```python
from build123d import *

# Parameters (mm, degrees)
F0_W     = 20.769432
F0_H     = 34.9758
F1_DEPTH = 2.54


with BuildPart() as f1:
    # F0 (on Front) → F1 (new body)
    with BuildSketch(Plane.XZ):
        Polygon((-12.7, 0), (0, 0), (12.7, 0), (12.7, 9.4996), (-12.7, 9.4996), align=None)
        Polygon((-12.7, 18.4404), (-12.7, 9.4996), (12.7, 9.4996), (12.7, 18.4404), (11.725585, 18.4404), (-11.725585, 18.4404), align=None)
        Polygon((-11.725585, 28.448), (-11.725585, 18.4404), (11.725585, 18.4404), (11.725585, 28.448), (10.384716, 28.448), (-10.384716, 28.448), align=None)
        with Locations((0, 45.9359)):
            Rectangle(F0_W, F0_H)
    extrude(amount=-F1_DEPTH)


solid = f1.part
```
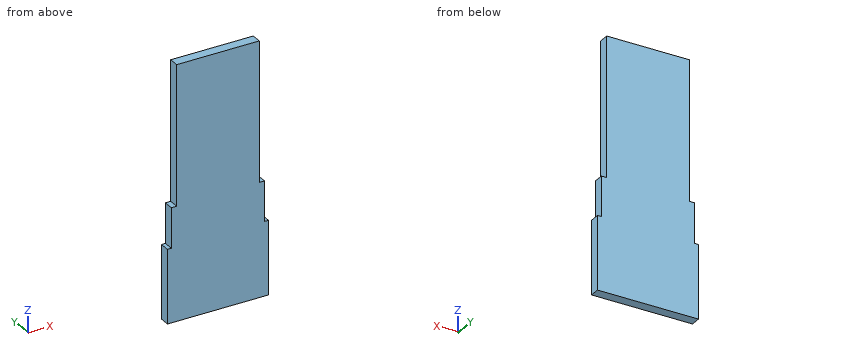
Verification items for the finished model (mm, model axes). Give positions to 0.01 mm unless a question says otherwise; leave off trailing zeros. Loops run counter-clockwise (first coordinate to the right, second up) from the corner with the lowest first, then second, coordinate; pieces in that order, holes last.
1. Section check A-A, the plane y = 1.1. Enter the section's corners in (x, z).
2. Thickness scan on line 1 (Z direction, x = 11.25, y = 0.2); line 2 (X direction, y = 1.25, z = 58.5); line 3 (X direction, y = 1.6, z = 22). Record the ranges inside material, lowest first.
3. Section check B-B, the plane z = 30.5. Enter the section's corners in (x, y), then the cut area to 3 significant figures.
4. Go/stop test with flat-tipped pins: pin 1 Ø1.1 at (x, y) = (-11, 2) entering from +Z; pin 2 Ø1.5 at (x, y) = (11, 1.5) entering from +Z; pin 3 Ø1.3 at (y, z) = (1, 25) entering from -X; pin 4 Ø1.3 at (y, z) = (1, 42) entering from -X. Record where each tip stops, or that it passes through.
Geometry says:
1. outline: (-12.7, 0) - (12.7, 0) - (12.7, 18.44) - (11.73, 18.44) - (11.73, 28.45) - (10.38, 28.45) - (10.38, 63.42) - (-10.38, 63.42) - (-10.38, 28.45) - (-11.73, 28.45) - (-11.73, 18.44) - (-12.7, 18.44) - close
2. line 1: z = 0 to 28.45
2. line 2: x = -10.38 to 10.38
2. line 3: x = -11.73 to 11.73
3. outline: (-10.38, 0) - (10.38, 0) - (10.38, 2.54) - (-10.38, 2.54) - close
3. area: 52.8 mm2
4. pin 1: stops at z = 28.45
4. pin 2: stops at z = 63.42
4. pin 3: stops at x = -11.73
4. pin 4: stops at x = -10.38
